Autodesk Inventor part; units mm, degrees
ref_plane "YZ Plane" through (0, 0, 0) normal (1, 0, 0) x (0, 1, 0)
ref_plane "XZ Plane" through (0, 0, 0) normal (0, 1, 0) x (-1, 0, 0)
ref_plane "XY Plane" through (0, 0, 0) normal (0, 0, 1) x (1, 0, 0)
sketch "Boceto1" plane through (0, 0, 0) normal (0, 1, 0) x (-1, 0, 0)
  circle A0 centre (0, 0) radius 1.45
  dimension "d3" = 2.9
extrude "Extrusión1" add sketch "Boceto1" along normal blind 25
sketch "Boceto3" plane through (0, 0, 0) normal (0, -1, 0) x (1, 0, 0)
  circle A0 centre (0, 0) radius 5
  dimension "d5" = 10
extrude "Extrusión2" add sketch "Boceto3" along normal blind 5.7
chamfer "Chaflán1" distance 0.6 angle 45 1 edges at (-5, 0, 0)
sketch "Boceto5" plane through (0, -5.7, 0) normal (0, -1, 0) x (1, 0, 0)
  line L0 (0, 0) -> (0, 5) construction
  line L1 (0, 0) -> (5, 0) construction
  line L2 (0, 0) -> (4.3301, -2.5) construction
  line L3 (0, 0) -> (5, 0) construction
  line L4 (0, 0) -> (2.5, -4.3301) construction
  line L5 (0, 0) -> (5, 0) construction
  line L6 (0, 0) -> (0, -5) construction
  line L7 (0, 0) -> (5, 0) construction
  line L8 (0, 0) -> (-5, 0) construction
  line L9 (0, 0) -> (-5, 0) construction
  line L10 (0, 0) -> (-4.3301, -2.5) construction
  line L11 (0, 0) -> (-2.5, -4.3301) construction
  line L12 (0, 0) -> (4.3301, 2.5) construction
  line L13 (0, 0) -> (2.5, 4.3301) construction
  line L14 (0, 0) -> (-4.3301, 2.5) construction
  line L15 (0, 0) -> (-2.5, 4.3301) construction
  line L16 (4.3301, -2.5) -> (2.5, -4.3301)
  line L17 (2.5, -4.3301) -> (0, -5)
  line L18 (0, -5) -> (-2.5, -4.3301)
  line L19 (-2.5, -4.3301) -> (-4.3301, -2.5)
  line L20 (-5, 0) -> (-4.3301, 2.5)
  line L21 (-4.3301, 2.5) -> (-2.5, 4.3301)
  line L22 (-2.5, 4.3301) -> (0, 5)
  line L23 (0, 5) -> (2.5, 4.3301)
  line L24 (2.5, 4.3301) -> (4.3301, 2.5)
  line L25 (4.3301, 2.5) -> (5, 0)
  line L26 (5, 0) -> (4.3301, -2.5)
  line L27 (-4.3301, -2.5) -> (-5, 0)
  circle A0 centre (0, 0) radius 5
  dimension "d13" = 5
  dimension "d14" = 30
  dimension "d16" = 60
extrude "Extrusión3" cut sketch "Boceto5" against normal blind 6 contours A0 L16 | L26 A0 | A0 L17 | L25 A0 | A0 L18 | L24 A0 | A0 L19 | L23 A0 | A0 L27 | L22 A0 | A0 L20 | L21 A0
sketch "Boceto7" plane through (0, 25, 0) normal (0, 1, 0) x (1, 0, 0)
  circle A0 centre (0, 0) radius 1.45
  dimension "d22" = 2.9
extrude "Extrusión5" cut sketch "Boceto7" against normal blind 29
sketch "Boceto8" plane through (0, -5.7, 0) normal (0, -1, 0) x (1, 0, 0)
  circle A0 centre (0, 0) radius 4.65
  dimension "d25" = 9.3
extrude "Extrusión6" cut sketch "Boceto8" against normal blind 4.3
thread "Rosca2"
properties part number "Cubierta" material "Aluminio 6061"
Input: part model. Units: mm. Frame: model coordinates. A direction names the side the tool comes from. Coordinates: 2 decimals unless noted, no trailing zeros. Write each loop counter-clockwise with the first axis right and the second up, starting at its lowest first coordinate (ties: lowest second). Pieces come first, ordered by that corner, then holes.
1) Set-up query: faces 1 (the flat face through (-4.66, -3.1, -1.27)), 2 (the cylindrical face through (2.5, -3.58, 3.92)). Return all of +Z, -Z, +X, -X, +Y, -Y with unobstructed straight access to the full face (end or side cutting, diameter ignored); none if empty.
2) Section A-A on y = -4.7. Output: boundary loops of the cut face in (x, z), and give its area (3 significant figures).
3) Material intervals for line 1 along Z through (x, y) = (0, -0.8); line 2 along Z through (x, y) = (0, -4.1), sorted ascending.
4) Section B-B on y = -1. Output: boundary loops of the cut face in (x, z), and give its area (3 significant figures).
5) Pin query (flat end, axial travel): pin 1 Ø1 at (x, z) = (-1.5, 2) entering from -Y; pin 2 Ø1.5 at (x, y) = (2, -5) entering from +Z; pin 3 Ø2.5 at (x, z) = (0, 0) entering from +Y; pin 4 Ø2 at (x, y) = (-4, -4.5) entering from +Z. Return the tip coordinate at first contact, or that it passes through.
6) Mould query, pull axis X, two halves, no side actions, for faces 3 (the flat face through (4.66, -3.1, 1.27)), 4 (the flat face through (2, 0, 0)), 5 (the cylindrical face through (-1.45, -0.69, -0.06)). Classes: pulls with the +X half, pulls with the -X half, needs draft (parallel to the pull), parting line crosses it, or undercut.
Check result:
1. face 1: -Z, -X, +Y, -Y
1. face 2: -Y
2. outline: (-5, 0) - (-4.33, -2.5) - (-2.5, -4.33) - (0, -5) - (2.5, -4.33) - (4.33, -2.5) - (5, 0) - (4.33, 2.5) - (2.5, 4.33) - (0, 5) - (-2.5, 4.33) - (-4.33, 2.5) - close; hole circle Ø9.3 at (0, 0)
2. area: 7.07 mm2
3. line 1: z = -5 to -1.45, 1.45 to 5
3. line 2: z = -5 to -4.65, 4.65 to 5
4. outline: (-5, 0) - (-4.33, -2.5) - (-2.5, -4.33) - (0, -5) - (2.5, -4.33) - (4.33, -2.5) - (5, 0) - (4.33, 2.5) - (2.5, 4.33) - (0, 5) - (-2.5, 4.33) - (-4.33, 2.5) - close; hole circle Ø2.9 at (0, 0)
4. area: 68.4 mm2
5. pin 1: stops at y = -1.4
5. pin 2: stops at z = 4.67
5. pin 3: passes through
5. pin 4: stops at z = 3.83
6. face 3: pulls with the +X half
6. face 4: needs draft
6. face 5: undercut
